Source: CAD feature listing. Evaluate the final solid. Frame: model axes, mm. A direction names the side the tool comes from. Give positions to 0.01 mm unless a question says otherwise; leave off trailing zeros. Put each result on its own line as item: value.
```python
from build123d import *

# Parameters (mm, degrees)
SKETCH_R           = 1.5
PAD_DEPTH          = 3
FILLET_R           = 0.5
POCKET_DEPTH       = 105.626533
FILLET001_R        = 0.3
POLARPATTERN_COUNT = 4
FILLET002_R        = 0.3
FILLET003_R        = 0.3
FILLET004_R        = 0.3


with BuildPart() as part:
    # Sketch → Pad (new body)
    with BuildSketch(Plane.XY):
        with BuildLine():
            Line((-13.555442, 8.5), (-3.039737, 22.6))
            ThreePointArc((3.039737, 22.6), (0, 24), (-3.039737, 22.6))
            Line((3.039737, 22.6), (13.555442, 8.5))
            ThreePointArc((-13.555442, 8.5), (0, -16), (13.555442, 8.5))
        make_face()
        with Locations((0, 20)):
            Circle(SKETCH_R, mode=Mode.SUBTRACT)
    extrude(amount=PAD_DEPTH)

    # Fillet
    fillet_edges = [part.edges().sort_by_distance(p)[0] for p in [
        (8.297589, 15.55, 3),
        (0, -16, 3),
        (-8.297589, 15.55, 3),
        (0, 24, 3),
        (-1.5, 20, 3),
    ]]
    fillet(fillet_edges, radius=FILLET_R)

    # Sketch001 (on Face6 of Pad) → Pocket (cut, through all)
    with BuildSketch(Plane(origin=(0, 0, 0), x_dir=(1, 0, 0), z_dir=(0, 0, -1))):
        with BuildLine():
            Line((-3, 4.94), (3, 4.94))
            Line((3, 4.94), (8.656854, 10.596854))
            ThreePointArc((8.656854, 10.596854), (6.496296, 12.042948), (4.101219, 13.054288))
            Line((4.101219, 13.054288), (0, 8.953069))
            Line((0, 8.953069), (-4.101219, 13.054288))
            ThreePointArc((-4.101219, 13.054288), (-6.496296, 12.042948), (-8.656854, 10.596854))
            Line((-8.656854, 10.596854), (-3, 4.94))
        make_face()
    pocket = extrude(amount=-POCKET_DEPTH, mode=Mode.SUBTRACT)

    # Fillet001
    fillet001_edges = [part.edges().sort_by_distance(p)[0] for p in [
        (-3, -4.94, 1.5),
        (3, -4.94, 1.5),
        (-8.656854, -10.596854, 1.5),
        (0, -8.953069, 1.5),
        (8.656854, -10.596854, 1.5),
        (4.101219, -13.054288, 1.5),
        (-4.101219, -13.054288, 1.5),
    ]]
    fillet(fillet001_edges, radius=FILLET001_R)

    # PolarPattern: Pocket ×4 about axis
    polarpattern_axis = Axis((0, 0, 0), (0, 0, -1))
    for i in range(1, POLARPATTERN_COUNT):
        add(pocket.rotate(polarpattern_axis, i * 360 / POLARPATTERN_COUNT), mode=Mode.SUBTRACT)

    # Fillet002
    fillet002_edges = [part.edges().sort_by_distance(p)[0] for p in [
        (10.596854, 8.656854, 1.5),
        (8.953069, 0, 1.5),
        (13.054288, 4.101219, 1.5),
        (13.054288, -4.101219, 1.5),
        (4.94, 3, 1.5),
        (4.94, -3, 1.5),
        (10.596854, -8.656854, 1.5),
    ]]
    fillet(fillet002_edges, radius=FILLET002_R)

    # Fillet003
    fillet003_edges = [part.edges().sort_by_distance(p)[0] for p in [
        (-10.596854, -8.656854, 1.5),
        (-8.953069, 0, 1.5),
        (-13.054288, 4.101219, 1.5),
        (-13.054288, -4.101219, 1.5),
        (-4.94, 3, 1.5),
        (-4.94, -3, 1.5),
        (-10.596854, 8.656854, 1.5),
    ]]
    fillet(fillet003_edges, radius=FILLET003_R)

    # Fillet004
    fillet004_edges = [part.edges().sort_by_distance(p)[0] for p in [
        (-8.656854, 10.596854, 1.5),
        (-3, 4.94, 1.5),
        (3, 4.94, 1.5),
        (8.656854, 10.596854, 1.5),
        (0, 8.953069, 1.5),
        (-4.101219, 13.054288, 1.5),
        (4.101219, 13.054288, 1.5),
    ]]
    fillet(fillet004_edges, radius=FILLET004_R)


solid = part.part
```
(1) Line query: probe 1 along Y at (x, z) = (0, 1.2); probe 2 along Y at (x, z) = (-3, 1.25); probe 3 along Y at (x, z) = (-7, 1.3). Output: solid intervals per line, ascending. Write a range as from..to.
Calculated:
probe 1: y = -16..-9.08, -4.94..4.94, 9.08..18.5, 21.5..24
probe 2: y = -15.72..-11.95, -4.97..4.97, 11.95..22.65
probe 3: y = -14.39..-11.76, -8.94..-5.06, 5.06..8.94, 11.76..17.29
(2) Section A-A on z = 1.55. Give the number of separate pieces and of enclosed holes in the cut face, then the cut area to 3 significant figures.
Calculated:
separate pieces: 1
enclosed holes: 5
area: 565 mm²
(3) First-contact query: P1, Ø1, axis at y = 6, z = 2, coming from the +X side (3 decimals); P2, Ø0.9, axis at y = 1, z = 1, coming from the -X side; P3, Ø1, axis at y = 16.5, z = 0.5, coming from the -X side. Flat tips, straight axial feed; report the tip coordinate or a pass-through.
Calculated:
P1: stops at x = 15.025
P2: stops at x = -15.99
P3: stops at x = -7.96
(4) Reachability of faces 1 (the flat face through (-8.37, 15.45, 1.23)), 2 (the flat face through (-5.72, 7.66, 1.48)) from +Z, -Z, +X, -X, +Y, -Y: full face, straight path, thin tool, end or side. Return the list, or none.
Calculated:
face 1: +Z, -Z, -X, +Y
face 2: +Z, -Z
(5) Draft query along Y for faces 3 (the flat face through (0, 0, 3)), 4 (the cylindrical face through (-8.11, 15.56, 2.85)), 5 (the flat face through (-11.071, -2.118, 1.479)), 6 (the cylindrical face through (6.457, -12.064, 1.479)). Return one class per face: released by +Y, released by -Y, zero draft, split by the parting line, or undercut.
Calculated:
face 3: zero draft
face 4: released by +Y
face 5: undercut
face 6: undercut
